For this review, use the dimensioned drawing (mm, ordinates from the lowest corner) and the shaded views. Coordinates: 2 decimals unless noted, no trailing zeros. Write each loop counter-clockwise with the first axis right and the second up, starting at its lowest first coordinate (ties: lowest second). Pieces come first, ordered by that corner, then holes. Notation, with made-up numbers: (47, 87.25) - (79, 87.25) arc R23 cw to (79, 111.25) - close; hole circle Ø4 at (35.5, 3). An arc over 180 degrees is marked (long way). Use one line per item in the form item = value. Start each with the question number.
1) For L1, parallel to Y at x = 9.5, z = 14; L2, parallel to X at y = 9.5, z = 6.75, list the stretches that pass through material, from the lowest coordinate up. Write a range as from..to.
2) We need section A-A (y = 9.5). Give the boundary of the cut face in (x, z), plus the area to 3 significant figures.
3) We need section B-B (x = 9.5). Give the boundary of the cut face in (y, z).
4) Insertion check: P1, Ø5.5, axis at y = 8.5, z = 2.5, coming from the -X side; P2, Ø2.5, axis at x = 1.5, y = 8.5, coming from the -Z side; P3, Ø5.5, axis at y = 12.5, z = 2, coming from the +X side. Each pin has a flat end and moves straight along its axis. Give the tip position at first contact, or say it passes through.
5) We need section C-C (z = 96.5). Give the boundary of the cut face in (x, y), plus the area to 3 significant figures.
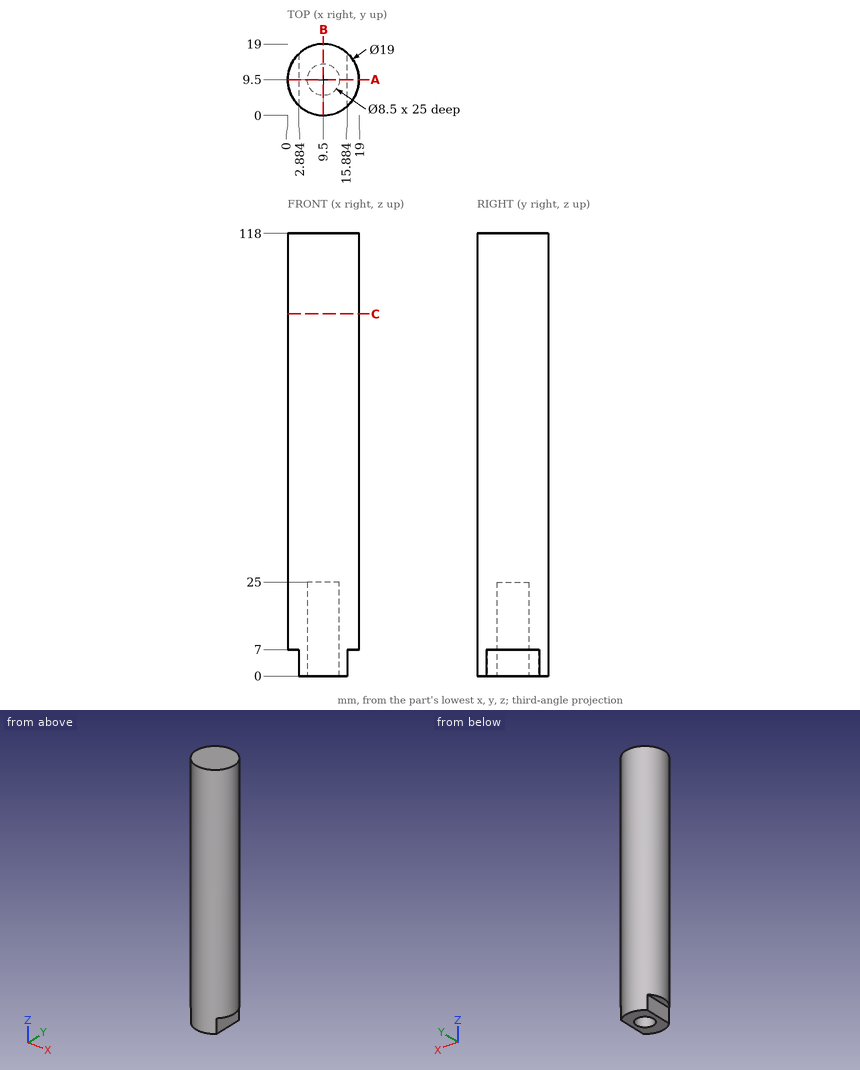
Determined:
q1.L1 = 0..5.25, 13.75..19
q1.L2 = 2.88..5.25, 13.75..15.88
q2.outline = (0, 7) - (2.88, 7) - (2.88, 0) - (5.25, 0) - (5.25, 25) - (13.75, 25) - (13.75, 0) - (15.88, 0) - (15.88, 7) - (19, 7) - (19, 118) - (0, 118) - close
q2.area = 1,990 mm²
q3.outline = (0, 0) - (5.25, 0) - (5.25, 25) - (13.75, 25) - (13.75, 0) - (19, 0) - (19, 118) - (0, 118) - close
q4.P1 = 2.88
q4.P2 = 7
q4.P3 = 15.88
q5.outline = circle Ø19 at (9.5, 9.5)
q5.area = 284 mm²
